Work out the finished part from the listing and answer in its coordinate system (mm). A direction names the side the tool comes from. Coordinates: 2 decimals unless noted, no trailing zeros. Loops run counter-clockwise (first coordinate to the right, second up) from the corner with the lowest first, then second, coordinate; pieces in that order, holes last. Notation, with made-up numbers: (53, 40) -> (89, 40) arc R21 cw to (89, 45) -> close; hole circle Ø1 at (-10.5, -0.5). An arc over 180 degrees is marked (long way). One line per question, with ' | ' between items.
```python
from build123d import *

# Parameters (mm, degrees)
BOSS_EXTRUDE1_DEPTH = 15
SKETCH2_W           = 32.3
SKETCH2_H           = 2.5
BOSS_EXTRUDE2_DEPTH = 23.5
SKETCH3_W           = 5
SKETCH3_H           = 6.2
CUT_EXTRUDE1_DEPTH  = 12.5
CUT_EXTRUDE2_REACH  = 28
SKETCH4_R           = 3.45
SKETCH5_R           = 1.2
CUT_EXTRUDE3_DEPTH  = 2.5
CUT_EXTRUDE4_REACH  = 39.3
SKETCH6_R           = 1.55
FILLET2_R           = 2
CUT_EXTRUDE6_REACH  = 4.5
SKETCH8_RX          = 9.634046057
SKETCH8_RY          = 6.312870092
SKETCH8_W           = 10.5
SKETCH8_H           = 3.175
SKETCH7_W           = 7.5
SKETCH7_H           = 7.5
SKETCH7_R           = 1.55
BOSS_EXTRUDE3_DEPTH = 1.25


with BuildPart() as part:
    # Sketch1 → Boss-Extrude1 (new body)
    with BuildSketch(Plane(origin=(0, 0, 0), x_dir=(1, 0, 0), z_dir=(0, 1, 0))):
        Polygon((0, 29.994099724), (-26, 29.994099724), (-26, -7.305900276), (0, -7.305900276), (0, -0.005900276), (-2.5, -0.005900276), (-2.5, -4.805900276), (-23.5, -4.805900276), (-23.5, 27.494099724), (-2.5, 27.494099724), (-2.5, 22.694099724), (0, 22.694099724), align=None)
    extrude(amount=BOSS_EXTRUDE1_DEPTH)

    # Sketch2 → Boss-Extrude2 (add, through all)
    with BuildSketch(Plane(origin=(-23.5, 0, 0), x_dir=(0, 0, -1), z_dir=(1, 0, 0))):
        with Locations((11.344099724, 1.25)):
            Rectangle(SKETCH2_W, SKETCH2_H)
    extrude(amount=BOSS_EXTRUDE2_DEPTH)

    # Sketch3 → Cut-Extrude1 (cut)
    with BuildSketch(Plane(origin=(0, 0, -29.994099724), x_dir=(-1, 0, 0), z_dir=(0, 0, -1))):
        with Locations((16.375, 8.6)):
            Rectangle(SKETCH3_W, SKETCH3_H)
    extrude(amount=-CUT_EXTRUDE1_DEPTH, mode=Mode.SUBTRACT)

    # Sketch4 → Cut-Extrude2 (cut, up to next)
    with BuildSketch(Plane.ZY.offset(26), mode=Mode.PRIVATE) as cut_extrude2_sk1:
        with Locations((-16.544099724, 8.6)):
            Circle(SKETCH4_R)
    cut_extrude2_tool1 = extrude(cut_extrude2_sk1.sketch, amount=-CUT_EXTRUDE2_REACH, mode=Mode.PRIVATE) & part.part
    add(cut_extrude2_tool1.solids().sort_by_distance((-26, 8.6, -16.5441))[0], mode=Mode.SUBTRACT)

    # Sketch5 → Cut-Extrude3 (cut)
    with BuildSketch(Plane(origin=(0, 0, 0), x_dir=(0, 0, -1), z_dir=(1, 0, 0))):
        with Locations((-2.555900276, 8.6)):
            Circle(SKETCH5_R)
    cut_extrude3 = extrude(amount=-CUT_EXTRUDE3_DEPTH, mode=Mode.SUBTRACT)

    # Mirror1: Cut-Extrude3 across plane
    add(cut_extrude3.mirror(Plane.XY.offset(-11.344099724)), mode=Mode.SUBTRACT)

    # Sketch6 → Cut-Extrude4 (cut, up to next)
    with BuildSketch(Plane.XY.offset(7.305900276), mode=Mode.PRIVATE) as cut_extrude4_sk1:
        with Locations((-13, 8.75)):
            Circle(SKETCH6_R)
    cut_extrude4_tool1 = extrude(cut_extrude4_sk1.sketch, amount=-CUT_EXTRUDE4_REACH, mode=Mode.PRIVATE) & part.part
    add(cut_extrude4_tool1.solids().sort_by_distance((-13, 8.75, 7.3059))[0], mode=Mode.SUBTRACT)

    # Fillet2
    fillet2_edges = [part.edges().sort_by_distance(p)[0] for p in [
        (0, 0, -11.344099724),
        (-13, 0, 7.305900276),
        (-26, 0, -11.344099724),
        (-13, 0, -29.994099724),
        (0, 7.5, 7.305900276),
        (-26, 7.5, 7.305900276),
        (-26, 7.5, -29.994099724),
        (0, 7.5, -29.994099724),
    ]]
    fillet(fillet2_edges, radius=FILLET2_R)

    # Sketch8 → Cut-Extrude6 (cut, up to next)
    with BuildSketch(Plane(origin=(0, 2.5, 0), x_dir=(1, 0, 0), z_dir=(0, 1, 0)), mode=Mode.PRIVATE) as cut_extrude6_sk1:
        with Locations(Location((-13, 11.344099724), (0, 0, 90))):
            Ellipse(SKETCH8_RX, SKETCH8_RY)
    cut_extrude6_tool1 = extrude(cut_extrude6_sk1.sketch, amount=-CUT_EXTRUDE6_REACH, mode=Mode.PRIVATE) & part.part
    add(cut_extrude6_tool1.solids().sort_by_distance((-13, 2.5, -11.3441))[0], mode=Mode.SUBTRACT)
    # Sketch8 → Cut-Extrude6 (cut, up to next)
    with BuildSketch(Plane(origin=(0, 2.5, 0), x_dir=(1, 0, 0), z_dir=(0, 1, 0)), mode=Mode.PRIVATE) as cut_extrude6_sk2:
        with Locations((-13, -2.231384095)):
            Rectangle(SKETCH8_W, SKETCH8_H)
    cut_extrude6_tool2 = extrude(cut_extrude6_sk2.sketch, amount=-CUT_EXTRUDE6_REACH, mode=Mode.PRIVATE) & part.part
    add(cut_extrude6_tool2.solids().sort_by_distance((-13, 2.5, 2.231384))[0], mode=Mode.SUBTRACT)
    # Sketch8 → Cut-Extrude6 (cut, up to next)
    with BuildSketch(Plane(origin=(0, 2.5, 0), x_dir=(1, 0, 0), z_dir=(0, 1, 0)), mode=Mode.PRIVATE) as cut_extrude6_sk3:
        with Locations((-13, 24.919583542)):
            Rectangle(SKETCH8_W, SKETCH8_H)
    cut_extrude6_tool3 = extrude(cut_extrude6_sk3.sketch, amount=-CUT_EXTRUDE6_REACH, mode=Mode.PRIVATE) & part.part
    add(cut_extrude6_tool3.solids().sort_by_distance((-13, 2.5, -24.919584))[0], mode=Mode.SUBTRACT)

    # Sketch7 → Boss-Extrude3 (add)
    with BuildSketch(Plane.XY.offset(7.305900276)):
        with Locations((-13, 8.75)):
            Rectangle(SKETCH7_W, SKETCH7_H)
        with Locations((-13, 8.75)):
            Circle(SKETCH7_R, mode=Mode.SUBTRACT)
    extrude(amount=BOSS_EXTRUDE3_DEPTH)


solid = part.part
```
1) Find section C-C (y = 6). Write down the section's boundary in (x, z) (3 decimals), plus the area to 3 significant figures.
Check values:
outline: (-26, -27.994) arc R2 ccw to (-24, -29.994) -> (-18.875, -29.994) -> (-18.875, -27.494) -> (-23.5, -27.494) -> (-23.5, -18.812) -> (-26, -18.812) -> close; (-26, -14.276) -> (-23.5, -14.276) -> (-23.5, 4.806) -> (-2.5, 4.806) -> (-2.5, 0.006) -> (0, 0.006) -> (0, 5.306) arc R2 ccw to (-2, 7.306) -> (-9.25, 7.306) -> (-9.25, 8.556) -> (-16.75, 8.556) -> (-16.75, 7.306) -> (-24, 7.306) arc R2 ccw to (-26, 5.306) -> close; (-13.875, -29.994) -> (-2, -29.994) arc R2 ccw to (0, -27.994) -> (0, -22.694) -> (-2.5, -22.694) -> (-2.5, -27.494) -> (-13.875, -27.494) -> close | area: 217 mm^2
2) Find the intervals of material crossed by line 1 along Z through (x, y) = (-2, 8.75); line 2 along Z through (x, y) = (-17.5, 4.5); line 3 along X through (y, z) = (8, 4), in increasing order.
Check values:
line 1: z = -29.99 to -26.43, -24.05 to -22.69, 0.01 to 1.37, 3.75 to 7.31 | line 2: z = -29.99 to -27.49, 4.81 to 7.31 | line 3: x = -26 to -23.5, -2.5 to 0
3) Flat-ended cylindrical pins translate along their axes: pin 1 (1.2 mm diameter, centred on x = -14.5, y = 1.5, fed in from +Z); pin 2 (6 mm diameter, centred on y = 8, z = -12.5, fed in from +X); pin 3 (0.8 mm diameter, centred on x = -1.5, y = 8.5, fed in from -Z). Find the tip coordinate at first contact, or state that the pin passes through.
Check values:
pin 1: stops at z = 7.31 | pin 2: stops at x = -23.5 | pin 3: stops at z = -29.99
4) The mould has two halves that part along Z. Classify faces 1 (the face through (-25.43, 8.591, 6.704)), 2 (the face through (-13, 1, -23.332)), 3 (the face through (-16, 5.5, -29)): released by +Z, released by -Z, zero draft, split by the parting line, or undercut.
Check values:
face 1: released by +Z | face 2: undercut | face 3: zero draft
5) Find section A-A (y = 4). Write down the section's boundary in (x, z), plus the area to 3 significant figures.
Check values:
outline: (-26, -27.99) arc R2 ccw to (-24, -29.99) -> (-2, -29.99) arc R2 ccw to (0, -27.99) -> (0, -22.69) -> (-2.5, -22.69) -> (-2.5, -27.49) -> (-23.5, -27.49) -> (-23.5, 4.81) -> (-2.5, 4.81) -> (-2.5, 0.01) -> (0, 0.01) -> (0, 5.31) arc R2 ccw to (-2, 7.31) -> (-24, 7.31) arc R2 ccw to (-26, 5.31) -> close | area: 231 mm^2
6) Find section B-B (x = -13). State how many separate pieces and enclosed holes the cut face has, plus the area to 3 significant figures.
Check values:
separate pieces: 5 | enclosed holes: 0 | area: 87.7 mm^2
7) Find section D-D (x = -4). Write down the section's boundary in (y, z), plus the area to 3 significant figures.
Check values:
outline: (0, -27.99) arc R2 ccw to (2, -29.99) -> (15, -29.99) -> (15, -27.49) -> (2.5, -27.49) -> (2.5, 4.81) -> (15, 4.81) -> (15, 7.31) -> (2, 7.31) arc R2 ccw to (0, 5.31) -> close | area: 154 mm^2
8) For faces 4 (the face through (-7.75, 1, -25)), 5 (the face through (-1.23, 8.96, -24.1)), 6 (the face through (-2.5, 9, 1)), 7 (the face through (-25.4, 0.57, -11.11)), 8 (the face through (-13.875, 9, -29)), determine the directions among +Z, -Z, +X, -X, +Y, -Y from which every point of the face is accessible in a straight line to the end or side of a thin tool.
Check values:
face 4: +Y, -Y | face 5: +X | face 6: +Y | face 7: +Z, -Z, -X, -Y | face 8: -Z
